Work out the finished part from the listing and answer in its coordinate system (mm). A direction names the side the tool comes from. Round coordinates to 2 decimals unless told otherwise and drop trailing zeros. Order: outer loops, then holes, each group sorted by start corner. A loop starts at its lowest first (then second) coordinate and runs counter-clockwise, first axis right, second up. Notation, with made-up numbers: (-31, 78.25) - (-8, 78.25) arc R17 cw to (-8, 109.25) - close; hole circle Ø11 at (72, 15.5). An arc over 180 degrees is marked (long way). Use CSV: the item, a comma, the result in double quotes.
Autodesk Inventor part; units mm, degrees
ref_plane "YZ Plane" through (0, 0, 0) normal (1, 0, 0) x (0, 1, 0)
ref_plane "XZ Plane" through (0, 0, 0) normal (0, 1, 0) x (-1, 0, 0)
ref_plane "XY Plane" through (0, 0, 0) normal (0, 0, 1) x (1, 0, 0)
sketch "Sketch1" plane through (0, 0, 0) normal (0, 0, 1) x (1, 0, 0)
  arc A0 (3.9123, 7.9106) -> (-5.3901, 7.9106) centre (-0.7389, 6.7419) ccw
  line L0 (3.9123, 7.9106) -> (-5.3901, 7.9106)
  line L1 (-5.3901, 7.9106) -> (3.9123, 7.9106)
  line L2 (3.9123, 7.9106) -> (3.9123, -0.326)
  line L3 (3.9123, -0.326) -> (-5.3901, -0.326)
  line L4 (-5.3901, -0.326) -> (-5.3901, 7.9106)
  point P0 (0, 0)
extrude "Extrusion1" add sketch "Sketch1" along normal blind 10
sketch "Sketch2" plane through (-5.3901, -0.326, 0) normal (0, -1, 0) x (1, 0, 0)
  circle A0 centre (5.3901, 5.2158) radius 2.2686
  point P0 (5.3901, 0)
extrude "Extrusion2" add sketch "Sketch2" along normal blind 10
properties part number "led"
(1) Find section A-A (x = -1.5). Determine the outline of the cut face in (y, z), and give its area (3 significant figures).
Findings below:
outline,"(-10.33, 3.51) - (-0.33, 3.51) - (-0.33, 0) - (11.48, 0) - (11.48, 10) - (-0.33, 10) - (-0.33, 6.92) - (-10.33, 6.92) - close"
area,"152 mm²"
(2) For faces 1 (the flat face through (-1, 6, 0)), 2 (the cylindrical face through (-0.49, -5.26, 7.43)), determine the directions among +Z, -Z, +X, -X, +Y, -Y from which every point of the face is accessible in a straight line to the end or side of a thin tool.
Findings below:
face 1,"-Z, +X, -X, +Y, -Y"
face 2,"-Y"
(3) Find section C-C (y = -3.5). Determine the outline of the cut face in (x, z), and give its area (3 significant figures).
Findings below:
outline,"circle Ø4.54 at (0, 5.22)"
area,"16.2 mm²"
(4) Each of these flat-tipped pins is pushed along its axis until it touches: pin 1 (2 mm diameter, centred on x = -2, y = 4.5, fed in from -Z); pin 2 (2 mm diameter, centred on x = 3, y = -8, fed in from +Z); pin 3 (4 mm diameter, centred on y = -8, z = 4.5, fed in from +X). Where does it stop, or does it pass through?
Findings below:
pin 1,"stops at z = 0"
pin 2,"stops at z = 6.29"
pin 3,"stops at x = 2.27"
(5) Find the intervals of material crossed by L1, parallel to Y at x = 2, z = 5.25; L2, parallel to Z at x = 1, y = -6; L3, parallel to Y at x = -2.75, z = 2.25, in increasing order. Write a range as from..to.
Findings below:
L1,"y = -10.33..10.68"
L2,"z = 3.18..7.25"
L3,"y = -0.33..11.1"
(6) Find section D-D (z = 9). Determine the outline of the cut face in (x, y).
Findings below:
outline,"(-5.39, -0.33) - (3.91, -0.33) - (3.91, 7.91) arc R4.8 ccw to (-5.39, 7.91) - close"
(7) Find section B-B (z = 6.5). Determine the outline of the cut face in (x, y).
Findings below:
outline,"(-5.39, -0.33) - (-1.87, -0.33) - (-1.87, -10.33) - (1.87, -10.33) - (1.87, -0.33) - (3.91, -0.33) - (3.91, 7.91) arc R4.8 ccw to (-5.39, 7.91) - close"
